Geometry check sheet. Reference: drawing and pictorial views, mm from the part's lowest x, y, z. A direction names the side the tool comes from. Give positions to 0.01 mm unless a question says otherwise; leave off trailing zeros. Write each loop counter-clockwise with the first axis right and the second up, starting at its lowest first coordinate (ties: lowest second). Pieces come first, ordered by that corner, then holes. Notation, with made-up numbers: (-17.75, 35.5) -> (18.25, 35.5) arc R18 ccw to (18.25, 49.5) -> close; hole circle Ø3 at (22.25, 17). An arc over 180 degrees is marked (long way). Use a Markdown table: item, result. Add a question column.
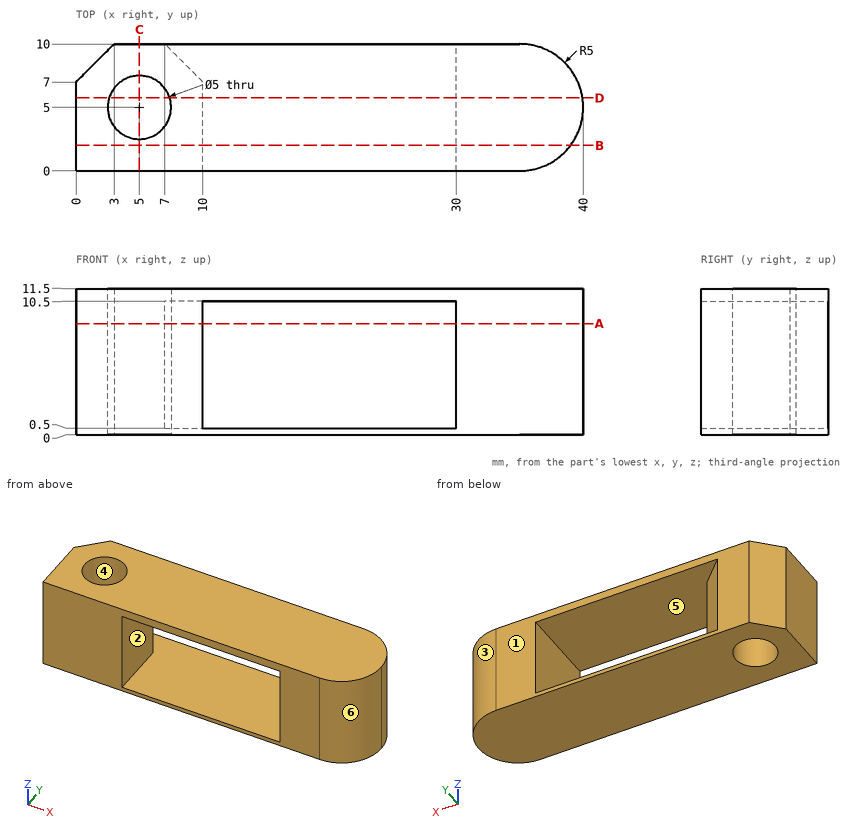
1) Sectioned sample at A-A, the plane z = 8.75. Count the separate pieces of the cut face and the enclosed holes in it, and give its area (3 significant figures).
2) Tool access check on the marked faces 1 and 2. Record the directions out of +Z, -Z, +X, -X, +Y, -Y that give a thin tool (end or side, any length) a straight path to the whole face; none if there is none.
3) Draft check along Y on the marked faces 3, 4, 5 and 6. Enter one of: +Y half, -Y half, draft (parallel to the pull), parting line (faces both ways), or undercut.
4) Gauge pin test, flat end, axial feed: P1, Ø1.5, axis at y = 2.5, z = 3.5, coming from the +X side. Record the tip position at first contact, or that the pin passes through.
5) Sectioned sample at B-B, the plane y = 2. Enter the section's corners in (x, z), and give its area (4 significant figures).
6) Sectioned sample at C-C, the plane x = 5. Enter the section's corners in (y, z).
7) Material ranges on probe 1 along Y at (x, z) = (5, 3.25); probe 2 along Z at (x, y) = (20, 5.5); probe 3 along X at (y, z) = (5.75, 9.75), recorded low to high. Write a range as [from, to].
8) Sectioned sample at D-D, the plane y = 5.75. Enter the section's corners in (x, z).
Check values:
| question | item | result |
|---|---|---|
| 1 | separate pieces | 2 |
| 1 | enclosed holes | 1 |
| 1 | area | 161 mm² |
| 2 | face 1 | +Z, -Z, +X, -X, +Y |
| 2 | face 2 | +Y, -Y |
| 3 | face 3 | +Y half |
| 3 | face 4 | undercut |
| 3 | face 5 | draft |
| 3 | face 6 | -Y half |
| 4 | P1 | x = 39.68 |
| 5 | outline | (0, 0) -> (39, 0) -> (39, 11.5) -> (0, 11.5) -> close; hole (10, 0.5) -> (30, 0.5) -> (30, 10.5) -> (10, 10.5) -> close |
| 5 | area | 248.5 mm² |
| 6 | outline | (0, 0) -> (2.5, 0) -> (2.5, 11.5) -> (0, 11.5) -> close; (7.5, 0) -> (10, 0) -> (10, 11.5) -> (7.5, 11.5) -> close |
| 7 | probe 1 | [0, 2.5], [7.5, 10] |
| 7 | probe 2 | [0, 0.5], [10.5, 11.5] |
| 7 | probe 3 | [0, 2.62], [7.38, 10], [30, 39.94] |
| 8 | outline | (0, 0) -> (2.62, 0) -> (2.62, 11.5) -> (0, 11.5) -> close; (7.38, 0) -> (39.94, 0) -> (39.94, 11.5) -> (7.38, 11.5) -> close; hole (10, 0.5) -> (30, 0.5) -> (30, 10.5) -> (10, 10.5) -> close |
